Build history of the part. All positions in model axes, mm. Round coordinates to 2 decimals unless told otherwise and drop trailing zeros. Write each loop counter-clockwise with the first axis right and the second up, starting at its lowest first coordinate (ties: lowest second). Pieces come first, ordered by that corner, then holes.
Item 1: Band-saw the part on B-B, the plane z = 0.7. Count the separate pieces of the cut face and the enclosed holes in it, then the cut area to 3 significant figures.
Item 2: Drop flat-ended pins along their axis: pin 1 Ø2 at (x, z) = (71.5, 2.5) entering from +Y; pin 2 Ø1.2 at (y, z) = (69.5, 1) entering from -X; pin 3 Ø2 at (x, z) = (38.5, 1) entering from +Y; pin 4 Ø10 at (x, y) = (77.5, 77.5) entering from +Z. Give the stop position or say it passes through.
Item 3: Wall check: probe 1 along Y at (x, z) = (45, 1.25); probe 2 along X at (y, z) = (27.5, 1.85); probe 3 along X at (y, z) = (49.5, 1.65). Give the ranges that are in metal, low to high.
Item 4: Band-saw the part on A-A, the plane y = 25. Write the cut outline in (x, z), then the cut area to 3 significant figures.
Item 5: Band-saw the part on D-D, the plane y = 76.5. Write the cut outline in (x, z), then the cut area to 3 significant figures.
Item 6: Band-saw the part on C-C, the plane x = 11.5. Write the cut outline in (y, z).
Item 7: Mould opens along Y. For faces 1 (the flat face through (72.5, 45, 2)), 2 (the flat face through (54, 46, 4)) say: +Y half, -Y half, draft (parallel to the pull), parting line (faces both ways), or undercut.
```python
from build123d import *

# Parameters (mm, degrees)
SKETCH1_R           = 45
SKETCH1_R_2         = 0.5
SKETCH1_R_3         = 4
SKETCH1_W           = 4
SKETCH1_H           = 14
BOSS_EXTRUDE1_DEPTH = 4


with BuildPart() as part:
    # Sketch1 → Boss-Extrude1 (new body)
    with BuildSketch(Plane.XY):
        with Locations((45, 45)):
            Circle(SKETCH1_R)
        with Locations((37.6, 45)):
            Circle(SKETCH1_R_2, mode=Mode.SUBTRACT)
        with Locations((52.4, 45)):
            Circle(SKETCH1_R_2, mode=Mode.SUBTRACT)
        with Locations((45.121025162, 37.600989734)):
            Circle(SKETCH1_R_2, mode=Mode.SUBTRACT)
        with Locations((45, 52.4)):
            Circle(SKETCH1_R_2, mode=Mode.SUBTRACT)
        with Locations((45, 45)):
            Circle(SKETCH1_R_3, mode=Mode.SUBTRACT)
        with Locations((19.5, 67)):
            Rectangle(SKETCH1_W, SKETCH1_H, mode=Mode.SUBTRACT)
        with Locations((70.5, 45)):
            Rectangle(SKETCH1_W, SKETCH1_H, mode=Mode.SUBTRACT)
        with Locations((70.5, 23)):
            Rectangle(SKETCH1_W, SKETCH1_H, mode=Mode.SUBTRACT)
        with Locations((19.5, 45)):
            Rectangle(SKETCH1_W, SKETCH1_H, mode=Mode.SUBTRACT)
        with Locations((19.5, 23)):
            Rectangle(SKETCH1_W, SKETCH1_H, mode=Mode.SUBTRACT)
        with Locations((70.5, 67)):
            Rectangle(SKETCH1_W, SKETCH1_H, mode=Mode.SUBTRACT)
    extrude(amount=BOSS_EXTRUDE1_DEPTH)


solid = part.part
```
Results:
1. separate pieces: 1
1. enclosed holes: 11
1. area: 5,970 mm2
2. pin 1: stops at y = 82.08
2. pin 2: stops at x = 6.87
2. pin 3: stops at y = 89.66
2. pin 4: stops at z = 4
3. probe 1: y = 0 to 37.12, 38.09 to 41, 49 to 51.9, 52.9 to 90
3. probe 2: x = 3.54 to 17.5, 21.5 to 68.5, 72.5 to 86.46
3. probe 3: x = 0.23 to 17.5, 21.5 to 68.5, 72.5 to 89.77
4. outline: (4.69, 0) - (17.5, 0) - (17.5, 4) - (4.69, 4) - close; (21.5, 0) - (68.5, 0) - (68.5, 4) - (21.5, 4) - close; (72.5, 0) - (85.31, 0) - (85.31, 4) - (72.5, 4) - close
4. area: 290 mm2
5. outline: (12.86, 0) - (77.14, 0) - (77.14, 4) - (12.86, 4) - close
5. area: 257 mm2
6. outline: (14.95, 0) - (75.05, 0) - (75.05, 4) - (14.95, 4) - close
7. face 1: undercut
7. face 2: draft
